from build123d import *

# Parameters (mm, degrees)
SKETCH2_W            = 650
SKETCH2_H            = 120
BASE_FLANGE1_DEPTH   = 2
EDGE_FLANGE1_START   = -60
EDGE_FLANGE1_DEPTH   = 120
EDGE_FLANGE1_2_DEPTH = 120
CUT_EXTRUDE1_DEPTH   = 2


# Read off the part's stored shape, not the designer's step: Edge-Flange1
# Sheet-metal steps are written as plain solids
with BuildPart() as part:
    # Sketch2 → Base-Flange1 (new body)
    with BuildSketch(Plane(origin=(0, 0, 0), x_dir=(0, 0, -1), z_dir=(1, 0, 0))):
        Rectangle(SKETCH2_W, SKETCH2_H)
    extrude(amount=BASE_FLANGE1_DEPTH)

    # Edge-Flange1 outline → Edge-Flange1 (cut)
    with BuildSketch(Plane(origin=(0, 0, 0), x_dir=(1, 0, 0), z_dir=(0, 1, 0)).offset(EDGE_FLANGE1_START)):
        with BuildLine():
            ThreePointArc((0, 320.978152936), (0.201203495, 322.230808162), (0.784572558, 323.357444083))
            Line((0.784572558, 323.357444083), (2, 325))
            Line((2, 325), (0, 325))
            Line((0, 325), (0, 320.978152936))
        make_face()
    extrude(amount=EDGE_FLANGE1_DEPTH, mode=Mode.SUBTRACT)

    # Edge-Flange1 2 outline → Edge-Flange1 2 (add)
    with BuildSketch(Plane(origin=(0, 0, 0), x_dir=(1, 0, 0), z_dir=(0, 1, 0)).offset(EDGE_FLANGE1_START)):
        with BuildLine():
            Line((297.411393376, 724.225585433), (2, 325))
            Line((2, 325), (2, 320.978152936))
            ThreePointArc((2, 320.978152936), (2.100601748, 321.604480549), (2.392286279, 322.167798509))
            Line((2.392286279, 322.167798509), (299.019107097, 723.035939859))
            Line((299.019107097, 723.035939859), (297.411393376, 724.225585433))
        make_face()
    extrude(amount=EDGE_FLANGE1_2_DEPTH)

    # Sketch10 → Cut-Extrude1 (cut)
    with BuildSketch(Plane.ZY):
        with BuildLine():
            Line((280, -25), (280, -40))
            ThreePointArc((280, -40), (275, -45), (270, -40))
            Line((270, -40), (270, -25))
            ThreePointArc((270, -25), (275, -20), (280, -25))
        make_face()
        with BuildLine():
            Line((250, -25), (250, -40))
            ThreePointArc((250, -40), (245, -45), (240, -40))
            Line((240, -40), (240, -25))
            ThreePointArc((240, -25), (245, -20), (250, -25))
        make_face()
        with BuildLine():
            Line((130, -25), (130, -40))
            ThreePointArc((130, -40), (125, -45), (120, -40))
            Line((120, -40), (120, -25))
            ThreePointArc((120, -25), (125, -20), (130, -25))
        make_face()
        with BuildLine():
            Line((100, -25), (100, -40))
            ThreePointArc((100, -40), (95, -45), (90, -40))
            Line((90, -40), (90, -25))
            ThreePointArc((90, -25), (95, -20), (100, -25))
        make_face()
    extrude(amount=-CUT_EXTRUDE1_DEPTH, mode=Mode.SUBTRACT)


solid = part.part
Design review of the part built by this model. Coordinates are the model's own, in mm. A direction names the side the tool comes from. Give positions to 0.01 mm unless a question says otherwise; leave off trailing zeros. Loops run counter-clockwise (first coordinate to the right, second up) from the corner with the lowest first, then second, coordinate; pieces in that order, holes last. Notation, with made-up numbers: (7, 71.25) - (31, 71.25) arc R27 ccw to (31, 102.25) - close; hole circle Ø7 at (-15.75, 19). An arc over 180 degrees is marked (long way). Write item = value, one per line.
1) To check wall thickness, follow line 1 (X direction, y = 36, z = 200); line 2 (Z direction, x = 222, y = -30); line 3 (Z direction, x = 195, y = -33). State the ranges of each line that lie inside material, in increasing order.
Result sheet:
line_1 = 0 to 2
line_2 = -622.31 to -618.95
line_3 = -585.82 to -582.46
2) Take a section at C-C on x = 89.5. State the section outline as (y, z) points, and give its area (3 significant figures).
Result sheet:
outline = (-60, -443.25) - (60, -443.25) - (60, -439.89) - (-60, -439.89) - close
area = 403 mm2
3) Clearance check with flat-ended pins moving along their axes: pin 1 Ø4 at (x, y) = (151.5, -26) entering from +Z; pin 2 Ø2 at (y, z) = (-25, -125.5) entering from +X; pin 3 Ø12 at (x, y) = (60, -24.5) entering from -Z. State where each tip first meets the part, or that it passes through.
Result sheet:
pin_1 = -520.97
pin_2 = 2
pin_3 = -411.49
4) Take a section at B-B on z = -53.5. State the section outline as (x, y) points, and give its area (3 significant figures).
Result sheet:
outline = (0, -60) - (2, -60) - (2, 60) - (0, 60) - close
area = 240 mm2
5) Tool access review of faces 1 (the face through (0, 1, 7)), 2 (the face through (2, 1, 7)): name each direction out of +Z, -Z, +X, -X, +Y, -Y from which nothing blocks a thin tool from reaching the whole face with its end or side.
Result sheet:
face_1 = +Z, -Z, -X, +Y, -Y
face_2 = +Z, +X, +Y, -Y
6) Take a section at A-A on y = 26. State the section outline as (x, z) points.
Result sheet:
outline = (0, -320.98) arc R4 ccw to (0.78, -323.36) - (297.41, -724.23) - (299.02, -723.04) - (2.39, -322.17) arc R2 cw to (2, -320.98) - (2, 325) - (0, 325) - close
